from build123d import *

# Parameters (mm, degrees)
SKETCH2_W           = 60
SKETCH2_H           = 5
BOSS_EXTRUDE1_DEPTH = 7
CUT_EXTRUDE1_DEPTH  = 12
SKETCH5_R           = 1.4
CUT_EXTRUDE2_DEPTH  = 3
FILLET1_R           = 10
FILLET2_R           = 0.3


with BuildPart() as part:
    # Sketch2 → Boss-Extrude1 (new body)
    with BuildSketch(Plane(origin=(0, 0, 0), x_dir=(1, 0, 0), z_dir=(0, 1, 0))):
        Polygon((-50.5, 5), (-30, 5), (-30, 0), (-30, -3), (-50.5, -3), align=None)
        with Locations((0, 2.5)):
            Rectangle(SKETCH2_W, SKETCH2_H)
        Polygon((30, -3), (30, 0), (30, 5), (50.5, 5), (50.5, -3), align=None)
    extrude(amount=BOSS_EXTRUDE1_DEPTH)

    # Sketch4 → Cut-Extrude1 (cut)
    with BuildSketch(Plane.XY.offset(3)):
        Polygon((-31.65, 2.9), (-31.65, 5.5), (-40.25, 5.5), (-48.85, 5.5), (-48.85, 2.9), align=None)
        Polygon((48.85, 2.9), (31.65, 2.9), (31.65, 5.5), (40.25, 5.5), (48.85, 5.5), align=None)
    extrude(amount=-CUT_EXTRUDE1_DEPTH, mode=Mode.SUBTRACT)

    # Sketch5 → Cut-Extrude2 (cut)
    with BuildSketch(Plane.XZ):
        with Locations(Location((40.25, -1, 0), (0, 0, 270))):
            Circle(SKETCH5_R)
        with Locations(Location((-40.25, -1, 0), (0, 0, 270))):
            Circle(SKETCH5_R)
    extrude(amount=-CUT_EXTRUDE2_DEPTH, mode=Mode.SUBTRACT)

    # Fillet1
    # the kernel refuses this fillet: 10 mm, written as the material it adds along each edge
    with BuildSketch(Plane(origin=(-30, 0, 0), x_dir=(0, 0, 1), z_dir=(0, 1, 0))) as fillet1_piece_1:
        with BuildLine():
            CenterArc((10, 7.141428429), FILLET1_R, 180, 45.572995999)
            Line((0, 7.141428429), (-0.2, 7.141428429))
            Line((-0.2, 7.141428429), (-0.2, 0))
            Line((-0.2, 0), (0, -0.2))
            ThreePointArc((0, -0.2), (1.5, -0.2), (2.86, -0.142828569))
            Line((2.86, -0.142828569), (3, 0))
        make_face()
    extrude(amount=7)
    with BuildSketch(Plane(origin=(30, 0, 0), x_dir=(0, 0, 1), z_dir=(0, 1, 0))) as fillet1_piece_2:
        with BuildLine():
            CenterArc((10, -7.141428429), FILLET1_R, 134.427004001, 45.572995999)
            Line((0, -7.141428429), (-0.2, -7.141428429))
            Line((-0.2, -7.141428429), (-0.2, 0))
            Line((-0.2, 0), (0, 0.2))
            ThreePointArc((0, 0.2), (1.5, 0.2), (2.86, 0.142828569))
            Line((2.86, 0.142828569), (3, 0))
        make_face()
    extrude(amount=7)

    # Fillet2
    fillet2_edges = [part.edges().sort_by_distance(p)[0] for p in [
        (40.25, 0, 0.4),
        (-40.25, 0, 0.4),
    ]]
    fillet(fillet2_edges, radius=FILLET2_R)


solid = part.part
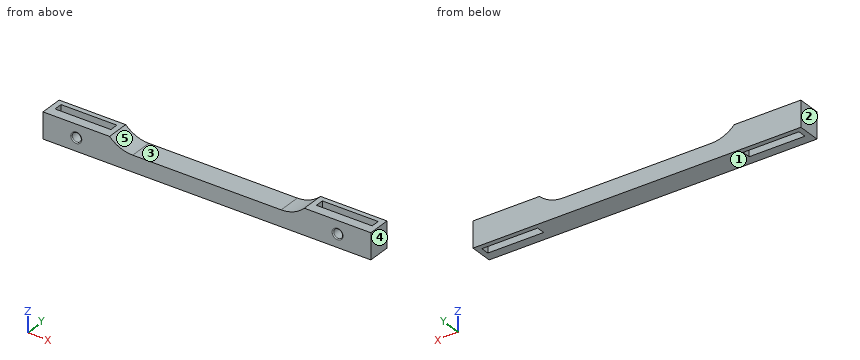
Could you check a few things on this model? Use its own coordinates, in mm. Face numbers are marked on the shaded views. A direction names the side the tool comes from. Round coordinates to 2 decimals unless told otherwise and drop trailing zeros. Order: outer loops, then holes, each group sorted by start corner. A loop starts at its lowest first (then second) coordinate and runs counter-clockwise, first axis right, second up.
Q1. Which directions (+Z, -Z, +X, -X, +Y, -Y) give clear straight access to the entire face, cutting with the end or side of a thin tool? Please do the marked faces 4 and 5.
Geometry says:
face 4: +Z, -Z, +X, +Y, -Y
face 5: +Z, +Y, -Y
Q2. I'm going to push flat-ended pins straight in: P1, Ø3.5, axis at x = 8, y = 2.5, coming from the +Z side; P2, Ø2, axis at x = -40.25, z = -1, coming from the -Y side. Where does each tip first touch, or does it pass through?
Geometry says:
P1: stops at z = 0
P2: stops at y = 5.5
Q3. Thinking about a two-plate mould opening in X: for the marked faces 1, 2 and 3, which applies, released by +X, released by -X, zero draft, split by the parting line, or undercut?
Geometry says:
face 1: zero draft
face 2: released by -X
face 3: undercut
Q4. Imagine slicing it at B-B, the plane z = -4. List the corners of the cut face in (x, y) for me, then the cut area to 3 significant figures.
Geometry says:
outline: (-50.5, 0) - (50.5, 0) - (50.5, 7) - (-50.5, 7) - close; hole (-48.85, 2.9) - (-31.65, 2.9) - (-31.65, 5.5) - (-48.85, 5.5) - close; hole (31.65, 2.9) - (48.85, 2.9) - (48.85, 5.5) - (31.65, 5.5) - close
area: 618 mm2
Q5. Please list where these lines run through material, in increasing order: probe 1 along X at (y, z) = (3.25, -0.25); probe 2 along X at (y, z) = (1.2, -1); probe 3 along Y at (x, z) = (33, -1).
Geometry says:
probe 1: x = -50.5 to -48.85, -31.65 to 31.65, 48.85 to 50.5
probe 2: x = -50.5 to -41.65, -38.85 to 38.85, 41.65 to 50.5
probe 3: y = 0 to 2.9, 5.5 to 7
Q6. Imagine slicing it at C-C, the plane y = 2. List the corners of the cut face in (x, z) for me, then the cut area to 3 significant figures.
Geometry says:
outline: (-50.5, -5) - (50.5, -5) - (50.5, 3) - (30, 3) arc R10 cw to (22.86, 0) - (-22.86, 0) arc R10 cw to (-30, 3) - (-50.5, 3) - close; hole circle Ø2.8 at (-40.25, -1); hole circle Ø2.8 at (40.25, -1)
area: 629 mm2
Q7. Imagine slicing it at A-A, the plane x = -40.25. List the corners of the cut face in (y, z) for me, then the cut area to 3 significant figures.
Geometry says:
outline: (0, -5) - (2.9, -5) - (2.9, -2.4) - (0.3, -2.4) arc R0.3 ccw to (0, -2.7) - close; (0, 0.7) arc R0.3 ccw to (0.3, 0.4) - (2.9, 0.4) - (2.9, 3) - (0, 3) - close; (5.5, -5) - (7, -5) - (7, 3) - (5.5, 3) - close
area: 27.0 mm2
